Could you check a few things on this model? Use its own coordinates, in mm. Round coordinates to 2 decimals unless told otherwise and drop trailing zeros. Loops run counter-clockwise (first coordinate to the right, second up) from the corner with the lowest first, then second, coordinate; pieces in that order, holes last.
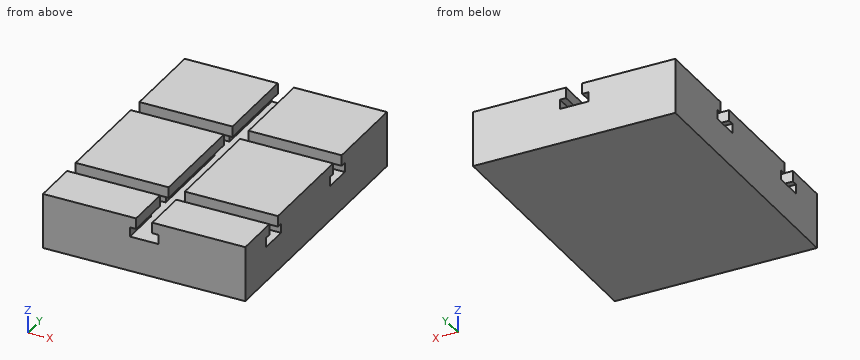
from build123d import *

# Parameters (mm, degrees)
F0_W     = 150
F0_H     = 41
F1_DEPTH = 100
F3_DEPTH = 200.001
F5_DEPTH = 150.001


with BuildPart() as f1:
    # F0 (on Front) → F1 (new body, symmetric)
    with BuildSketch(Plane.XZ):
        with Locations((0, -20.5)):
            Rectangle(F0_W, F0_H)
    extrude(amount=F1_DEPTH, both=True)

    # F2 (on face) → F3 (cut, through all)
    with BuildSketch(Plane.XZ.offset(100)):
        Polygon((6, 0), (-6, 0), (-6, -8), (-10.5, -8), (-10.5, -15), (10.5, -15), (10.5, -8), (6, -8), align=None)
    extrude(amount=-F3_DEPTH, mode=Mode.SUBTRACT)

    # F4 (on face) → F5 (cut, through all)
    with BuildSketch(Plane.YZ.offset(75)):
        Polygon((-54, 0), (-66, 0), (-66, -8), (-70.5, -8), (-70.5, -15), (-49.5, -15), (-49.5, -8), (-54, -8), align=None)
        Polygon((36, 0), (24, 0), (24, -8), (19.5, -8), (19.5, -15), (40.5, -15), (40.5, -8), (36, -8), align=None)
    extrude(amount=-F5_DEPTH, mode=Mode.SUBTRACT)


solid = f1.part
Item 1: If we section it at D-D, the plane y = 27: Please give me the cut outline in (x, z), then the cut area to 3 significant figures.
Results list:
outline: (-75, -41) - (75, -41) - (75, -15) - (-75, -15) - close
area: 3,900 mm2
Item 2: If we section it at A-A, the plane z = -2.5: Please give me the cut outline in (x, y), then the cut area to 3 significant figures.
Results list:
outline: (-75, -100) - (-6, -100) - (-6, -66) - (-75, -66) - close; (-75, -54) - (-6, -54) - (-6, 24) - (-75, 24) - close; (-75, 36) - (-6, 36) - (-6, 100) - (-75, 100) - close; (6, -100) - (75, -100) - (75, -66) - (6, -66) - close; (6, -54) - (75, -54) - (75, 24) - (6, 24) - close; (6, 36) - (75, 36) - (75, 100) - (6, 100) - close
area: 24,300 mm2
Item 3: If we section it at C-C, the plane y = -25.5: Please give me the cut outline in (x, z).
Results list:
outline: (-75, -41) - (75, -41) - (75, 0) - (6, 0) - (6, -8) - (10.5, -8) - (10.5, -15) - (-10.5, -15) - (-10.5, -8) - (-6, -8) - (-6, 0) - (-75, 0) - close
Item 4: If we section it at B-B, the plane x = 23.5: Please give me the cut outline in (y, z).
Results list:
outline: (-100, -41) - (100, -41) - (100, 0) - (36, 0) - (36, -8) - (40.5, -8) - (40.5, -15) - (19.5, -15) - (19.5, -8) - (24, -8) - (24, 0) - (-54, 0) - (-54, -8) - (-49.5, -8) - (-49.5, -15) - (-70.5, -15) - (-70.5, -8) - (-66, -8) - (-66, 0) - (-100, 0) - close
Item 5: If I drill on line 1 along Y through (x, z) = (41.5, -10); line 2 along Y through (x, z) = (52.5, -4.5); line 3 along Z through (x, y) = (8, -85), over which ranges is the centre line in solid material (lowest first)?
Results list:
line 1: y = -100 to -70.5, -49.5 to 19.5, 40.5 to 100
line 2: y = -100 to -66, -54 to 24, 36 to 100
line 3: z = -41 to -15, -8 to 0
Item 6: Will this pin go through, and if not, where does the flat tip stop? pin 1 (1.5 mm diameter, centred on x = -50, y = -60.5, fed in from +Z).
Results list:
pin 1: stops at z = -15
